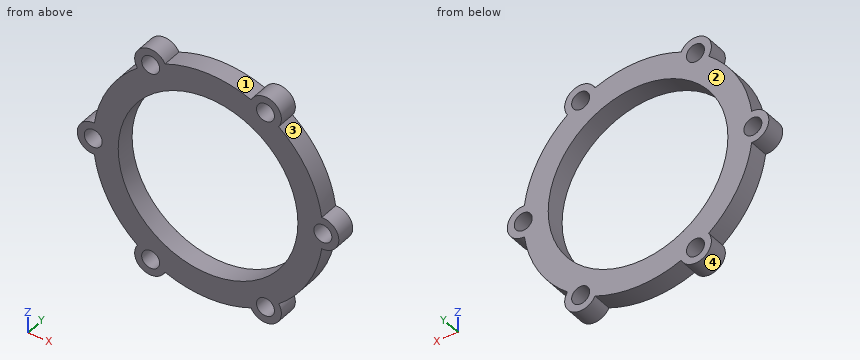
```python
from build123d import *

# Parameters (mm, degrees)
SKETCH2_R           = 45
SKETCH2_R_2         = 4.5
BOSS_EXTRUDE1_DEPTH = 10


with BuildPart() as part:
    # Sketch2 → Boss-Extrude1 (new body)
    with BuildSketch(Plane(origin=(0, 0, 0), x_dir=(1, 0, 0), z_dir=(0, 1, 0))):
        with BuildLine():
            ThreePointArc((56.943478261, 7.980619246), (49.796460718, 28.75), (35.383158136, 45.324189131))
            ThreePointArc((35.383158136, 45.324189131), (32.75, 56.724663948), (21.560320125, 53.304808377))
            ThreePointArc((21.560320125, 53.304808377), (0, 57.5), (-21.560320125, 53.304808377))
            ThreePointArc((-21.560320125, 53.304808377), (-32.75, 56.724663948), (-35.383158136, 45.324189131))
            ThreePointArc((-35.383158136, 45.324189131), (-49.796460718, 28.75), (-56.943478261, 7.980619246))
            ThreePointArc((-56.943478261, 7.980619246), (-65.5, 0), (-56.943478261, -7.980619246))
            ThreePointArc((-56.943478261, -7.980619246), (-49.796460718, -28.75), (-35.383158136, -45.324189131))
            ThreePointArc((-35.383158136, -45.324189131), (-32.75, -56.724663948), (-21.560320125, -53.304808377))
            ThreePointArc((-21.560320125, -53.304808377), (0, -57.5), (21.560320125, -53.304808377))
            ThreePointArc((21.560320125, -53.304808377), (32.75, -56.724663948), (35.383158136, -45.324189131))
            ThreePointArc((35.383158136, -45.324189131), (49.796460718, -28.75), (56.943478261, -7.980619246))
            ThreePointArc((56.943478261, -7.980619246), (65.5, 0), (56.943478261, 7.980619246))
        make_face()
        Circle(SKETCH2_R, mode=Mode.SUBTRACT)
        with Locations((28.75, 49.796460718)):
            Circle(SKETCH2_R_2, mode=Mode.SUBTRACT)
        with Locations((-28.75, 49.796460718)):
            Circle(SKETCH2_R_2, mode=Mode.SUBTRACT)
        with Locations((57.5, 0)):
            Circle(SKETCH2_R_2, mode=Mode.SUBTRACT)
        with Locations((-57.5, 0)):
            Circle(SKETCH2_R_2, mode=Mode.SUBTRACT)
        with Locations((28.75, -49.796460718)):
            Circle(SKETCH2_R_2, mode=Mode.SUBTRACT)
        with Locations((-28.75, -49.796460718)):
            Circle(SKETCH2_R_2, mode=Mode.SUBTRACT)
    extrude(amount=BOSS_EXTRUDE1_DEPTH)


solid = part.part
```
The model under review builds one solid part; all positions refer to its coordinate system, in mm. Face numbers are marked on the shaded views. Coordinates: 2 decimals unless noted, no trailing zeros. Write each loop counter-clockwise with the first axis right and the second up, starting at its lowest first coordinate (ties: lowest second). Pieces come first, ordered by that corner, then holes. Notation, with made-up numbers: (-1.5, 73) - (4.5, 73) arc R27 cw to (4.5, 106) - close; hole circle Ø8 at (29.25, 2). An arc over 180 degrees is marked (long way). Answer in a Markdown table with one row per item. Add a question column.
Q1. Consider section C-C on z = -20.5. Give the boundary of the cut face in (x, y), then the cut area to 3 significant figures.
Q2. Consider section A-A on x = 0. Give the boundary of the cut face in (y, z), then the cut area to 3 significant figures.
Q3. To check wall thickness, follow line 1 along Z through (x, y) = (-35.5, 3.25); line 2 along Z through (x, y) = (28.75, 3); line 3 along X through (y, z) = (6.5, -6.5). State the ranges of each line that lie inside material, in increasing order. Write a range as from..to.
Q4. Consider section D-D on x = -28.75. Give the boundary of the cut face in (y, z), then the cut area to 3 significant figures.
Q5. Consider section B-B on z = 0. Give the boundary of the cut face in (x, y), then the cut area to 3 significant figures.
Q6. Draft analysis for pull direction X (two halves, no side actions). For the marked faces 1, 2, 3 and 4, state which applies: +X half, -X half, draft (parallel to the pull), parting line (faces both ways), or undercut.
Q7. Clearance check with flat-ended pins moving along their axes: pin 1 (5 mm diameter, centred on x = 43.5, y = 6.5, fed in from +Z); pin 2 (2 mm diameter, centred on x = -18, y = 2, fed in from +Z); pin 3 (2 mm diameter, centred on x = 21, y = 2, fed in from +Z). State where each tip first meets the part, or that it passes through.
Answers below:
| question | item | result |
|---|---|---|
| 1 | outline | (-53.72, 0) - (-40.06, 0) - (-40.06, 10) - (-53.72, 10) - close; (40.06, 0) - (53.72, 0) - (53.72, 10) - (40.06, 10) - close |
| 1 | area | 273 mm² |
| 2 | outline | (0, -57.5) - (10, -57.5) - (10, -45) - (0, -45) - close; (0, 45) - (10, 45) - (10, 57.5) - (0, 57.5) - close |
| 2 | area | 250 mm² |
| 3 | line 1 | -54.09..-45.5, -45.23..-27.65, 27.65..45.23, 45.5..54.09 |
| 3 | line 2 | -57.8..-54.3, -45.3..-34.62, 34.62..45.3, 54.3..57.8 |
| 3 | line 3 | -62.16..-44.53, 44.53..62.16 |
| 4 | outline | (0, -57.8) - (10, -57.8) - (10, -54.3) - (0, -54.3) - close; (0, -45.3) - (10, -45.3) - (10, -34.62) - (0, -34.62) - close; (0, 34.62) - (10, 34.62) - (10, 45.3) - (0, 45.3) - close; (0, 54.3) - (10, 54.3) - (10, 57.8) - (0, 57.8) - close |
| 4 | area | 284 mm² |
| 5 | outline | (-65.5, 0) - (-62, 0) - (-62, 10) - (-65.5, 10) - close; (-53, 0) - (-45, 0) - (-45, 10) - (-53, 10) - close; (45, 0) - (53, 0) - (53, 10) - (45, 10) - close; (62, 0) - (65.5, 0) - (65.5, 10) - (62, 10) - close |
| 5 | area | 230 mm² |
| 6 | face 1 | undercut |
| 6 | face 2 | draft |
| 6 | face 3 | +X half |
| 6 | face 4 | undercut |
| 7 | pin 1 | z = 40.31 |
| 7 | pin 2 | z = 54.93 |
| 7 | pin 3 | z = 54.09 |
